from build123d import *

# Parameters (mm, degrees)
SKETCH1_W           = 180
SKETCH1_H           = 74.4
SKETCH1_R           = 1.6
SKETCH1_W_2         = 25
SKETCH1_H_2         = 6.2
BOSS_EXTRUDE1_DEPTH = 6


with BuildPart() as part:
    # Sketch1 → Boss-Extrude1 (new body)
    with BuildSketch(Plane(origin=(0, 0, 0), x_dir=(0, 0, -1), z_dir=(1, 0, 0))):
        Rectangle(SKETCH1_W, SKETCH1_H)
        with Locations((-41.666666667, -28.1)):
            Circle(SKETCH1_R, mode=Mode.SUBTRACT)
        with Locations((0, -28.1)):
            Circle(SKETCH1_R, mode=Mode.SUBTRACT)
        with Locations((-41.666666667, 28.1)):
            Circle(SKETCH1_R, mode=Mode.SUBTRACT)
        with Locations((0, 28.1)):
            Circle(SKETCH1_R, mode=Mode.SUBTRACT)
        with Locations(Location((41.666666667, 28.1, 0), (0, 0, 180))):
            Circle(SKETCH1_R, mode=Mode.SUBTRACT)
        with Locations((-20.833333333, -28.1)):
            Rectangle(SKETCH1_W_2, SKETCH1_H_2, mode=Mode.SUBTRACT)
        with Locations((-62.5, -28.1)):
            Rectangle(SKETCH1_W_2, SKETCH1_H_2, mode=Mode.SUBTRACT)
        with Locations((20.833333333, -28.1)):
            Rectangle(SKETCH1_W_2, SKETCH1_H_2, mode=Mode.SUBTRACT)
        with Locations((62.5, -28.1)):
            Rectangle(SKETCH1_W_2, SKETCH1_H_2, mode=Mode.SUBTRACT)
        with Locations((-62.5, 28.1)):
            Rectangle(SKETCH1_W_2, SKETCH1_H_2, mode=Mode.SUBTRACT)
        with Locations((-20.833333333, 28.1)):
            Rectangle(SKETCH1_W_2, SKETCH1_H_2, mode=Mode.SUBTRACT)
        with Locations((20.833333333, 28.1)):
            Rectangle(SKETCH1_W_2, SKETCH1_H_2, mode=Mode.SUBTRACT)
        with Locations((62.5, 28.1)):
            Rectangle(SKETCH1_W_2, SKETCH1_H_2, mode=Mode.SUBTRACT)
    extrude(amount=BOSS_EXTRUDE1_DEPTH)


solid = part.part
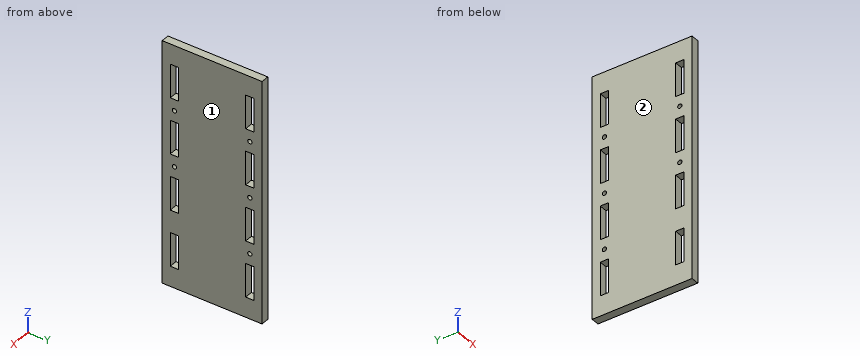
Build history of the part. All positions in model axes, mm. Face numbers are marked on the shaded views. Round coordinates to 2 decimals unless told otherwise and drop trailing zeros. Order: outer loops, then holes, each group sorted by start corner. A loop starts at its lowest first (then second) coordinate and runs counter-clockwise, first axis right, second up. Notation, with made-up numbers: M 44.25,19 L 85.25,19 A21 cw 85.25,47 Z; hole C 46,84.25 d3. An arc over 180 degrees is marked long. Use CSV: the item, a comma, the result in double quotes. Start each with the question number.
(1) Cut at A-A on y = -28.1. List the corners of the cut face in (x, z).
(2) Drill centre lines: probe 1 along Y at (x, z) = (2.3, -13); probe 2 along Z at (x, y) = (1.6, 31); probe 3 along Y at (x, z) = (2.6, 0). Where is each one in solid material? Low to high.
(3) Mould opens along X. For the marked faces 1 and 2 say: +X half, -X half, draft (parallel to the pull), parting line (faces both ways), or undercut.
(4) Cut at B-B on z = 0. List the corners of the cut face in (x, y), then the cut area to 3 significant figures.
(5) Cut at C-C on y = 28.1. State how many separate pieces and enclosed holes the cut face has, then the cut area to 3 significant figures.
Findings:
1,outline,"M 0,-90 L 6,-90 L 6,-75 L 0,-75 Z; M 0,-50 L 6,-50 L 6,-33.33 L 0,-33.33 Z; M 0,-8.33 L 6,-8.33 L 6,-1.6 L 0,-1.6 Z; M 0,1.6 L 6,1.6 L 6,8.33 L 0,8.33 Z; M 0,33.33 L 6,33.33 L 6,40.07 L 0,40.07 Z; M 0,43.27 L 6,43.27 L 6,50 L 0,50 Z; M 0,75 L 6,75 L 6,90 L 0,90 Z"
2,probe 1,"y = -37.2 to -31.2, -25 to 25, 31.2 to 37.2"
2,probe 2,"z = -90 to -75, -50 to -33.33, -8.33 to 8.33, 33.33 to 50, 75 to 90"
2,probe 3,"y = -37.2 to -29.7, -26.5 to 26.5, 29.7 to 37.2"
3,face 1,"+X half"
3,face 2,"-X half"
4,outline,"M 0,-37.2 L 6,-37.2 L 6,-29.7 L 0,-29.7 Z; M 0,-26.5 L 6,-26.5 L 6,26.5 L 0,26.5 Z; M 0,29.7 L 6,29.7 L 6,37.2 L 0,37.2 Z"
4,area,"408 mm^2"
5,separate pieces,"8"
5,enclosed holes,"0"
5,area,"422 mm^2"
